Autodesk Inventor part; units mm, degrees
ref_plane "YZ Plane" through (0, 0, 0) normal (1, 0, 0) x (0, 1, 0)
ref_plane "XZ Plane" through (0, 0, 0) normal (0, 1, 0) x (-1, 0, 0)
ref_plane "XY Plane" through (0, 0, 0) normal (0, 0, 1) x (1, 0, 0)
sketch "Sketch1" plane through (0, 0, 0) normal (0, 0, 1) x (1, 0, 0)
  circle A0 centre (0, 0) radius 20
  circle A1 centre (0, 0) radius 23
  dimension "d0" = 40
  dimension "d1" = 46
extrude "Extrusion1" add sketch "Sketch1" along normal mid plane 228
sketch "Sketch2" plane through (0, 0, 0) normal (1, 0, 0) x (0, 1, 0)
  line L0 (0, 70) -> (0, -70)
  line L1 (-70, 0) -> (70, 0)
  point P0 (0, 0)
  point P1 (0, 50)
  point P2 (0, -50)
  dimension "d19" = 50
  dimension "d20" = 100
hole "Hole1" at (0, 0, 50) at (0, 0, -50) direction (-1, 0, 0) diameter 4.5 end through all
sketch "Sketch3" plane through (0, 0, 0) normal (1, 0, 0) x (0, 1, 0)
  line L0 (23, -114) -> (7, -114)
  line L1 (7, -114) -> (7, 114)
  line L2 (7, 114) -> (23, 114)
  line L3 (23, 114) -> (23, -114)
  line L4 (23, 114) -> (-23, 114)
  line L5 (-23, -114) -> (23, -114)
  line L6 (0, 160.3) -> (0, -160.3)
  point P0 (0, 0)
  dimension "d13" = 0
  dimension "d14" = 0
  dimension "d15" = 7
extrude "Extrusion2" cut sketch "Sketch3" along normal through all both and the other way through all contours L0 L1 L2 L3
properties part number "Top_Tilt Pipe_4 Lanes" material "PVC-Piping"
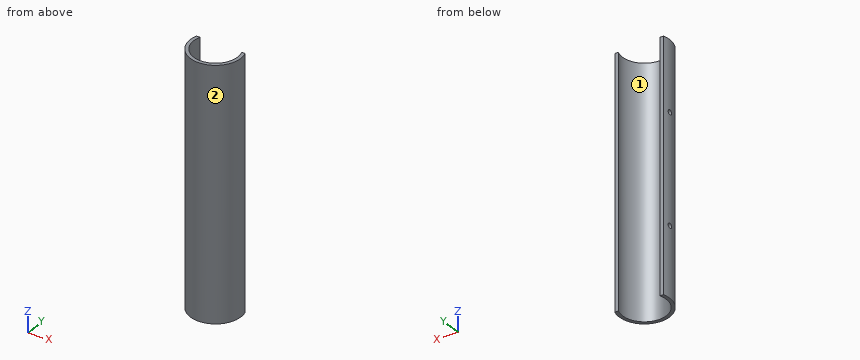
Model file for the job. Use its own axes, mm. Face numbers are marked on the shaded views. Coordinates: 2 decimals unless noted, no trailing zeros. Write each loop counter-clockwise with the first axis right and the second up, starting at its lowest first coordinate (ties: lowest second). Pieces come first, ordered by that corner, then holes. Notation, with made-up numbers: (80, 55) -> (86, 55) arc R36 cw to (86, 93) -> close; hole circle Ø5 at (-16.75, 42). An arc over 180 degrees is marked (long way). One line per item, written item: value. Start each with the question number.
1) Slice it at A-A on y = 0. Write the cut outline in (x, z), then the cut area to 3 significant figures.
2) Flat gauge pins, fed straight in: pin 1 Ø5 at (y, z) = (-14, -60) entering from -X; pin 2 Ø12 at (y, z) = (-9, -65) entering from +X; pin 3 Ø4 at (x, z) = (10, 57) entering from -Y. Where does each tip first touch, or does it go through?
3) Probe probe 1 along Z at (x, y) = (-21, 0); probe 2 along X at (y, z) = (0, 53.5); probe 3 along X at (y, z) = (-5.5, -71). List the from-to ranges inside material, lowest first.
4) Slice it at B-B on y = -12. Write the cut outline in (x, z).
5) Slice it at C-C on z = -50. Write the cut outline in (x, y) (3 decimals).
6) Slice it at D-D on x = 0. Write the cut outline in (y, z).
7) Pull direction Y, two halves, no side cores. Call the marked faces 1 and 2: +Y half, -Y half, draft (parallel to the pull), parting line (faces both ways), or undercut.
Answers follow:
1. outline: (-23, -114) -> (-20, -114) -> (-20, -52.25) -> (-23, -52.25) -> close; (-23, -47.75) -> (-20, -47.75) -> (-20, 47.75) -> (-23, 47.75) -> close; (-23, 52.25) -> (-20, 52.25) -> (-20, 114) -> (-23, 114) -> close; (20, -114) -> (23, -114) -> (23, 114) -> (20, 114) -> close
1. area: 1,340 mm2
2. pin 1: x = -19.92
2. pin 2: x = 22.8
2. pin 3: y = -21.56
3. probe 1: -114 to -52.25, -47.75 to 47.75, 52.25 to 114
3. probe 2: -23 to -20, 20 to 23
3. probe 3: -22.33 to -19.23, 19.23 to 22.33
4. outline: (-19.62, -114) -> (-16, -114) -> (-16, 114) -> (-19.62, 114) -> close; (16, -114) -> (19.62, -114) -> (19.62, 114) -> (16, 114) -> close
5. outline: (-22.89, -2.25) arc R23 ccw (long way) to (21.909, 7) -> (18.735, 7) arc R20 cw (long way) to (-19.873, -2.25) -> close; (-22.89, 2.25) -> (-19.873, 2.25) arc R20 cw to (-18.735, 7) -> (-21.909, 7) arc R23 ccw to start
6. outline: (-23, -114) -> (-20, -114) -> (-20, 114) -> (-23, 114) -> close
7. face 1: undercut
7. face 2: parting line
